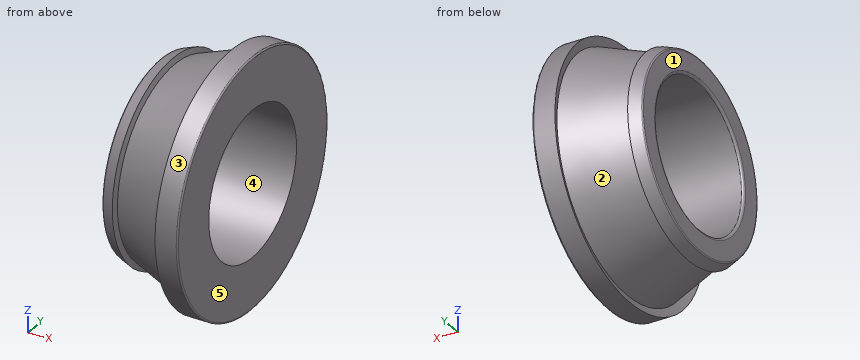
Solid Edge part; units mm, degrees
sketch "Sketch1" plane through (0, 0, 0) normal (0, 0, 1) x (1, 0, 0)
  arc A0 (0, 15.5) -> (0.5, 15) centre (0.5, 15.5) ccw
  line L0 (0.5, 15) -> (19, 15)
  line L1 (19, 15) -> (19, 25.318)
  arc A1 (19, 25.318) -> (18.711, 25.607) centre (18.711, 25.318) ccw
  line L2 (18.711, 25.607) -> (14.373, 25.607)
  line L3 (14.373, 25.607) -> (15.0184, 23.853)
  line L4 (15.0184, 23.853) -> (2.95, 19.4124)
  line L5 (2.95, 19.4124) -> (2.5514, 20.4958)
  line L6 (2.5514, 20.4958) -> (0.1964, 19.6293)
  arc A2 (0.1964, 19.6293) -> (0, 19.3477) centre (0.3, 19.3477) ccw
  line L7 (0, 19.3477) -> (0, 15.5)
revolve "RevolvedProtrusion1" add sketch "Sketch1" angle 360 about axis through (50, 0, 0) along (-1, 0, 0)
Geometry check sheet. Reference: the model listing, model coordinates, mm. Face numbers are marked on the shaded views. A direction names the side the tool comes from. Coordinates: 2 decimals unless noted, no trailing zeros. Order: outer loops, then holes, each group sorted by start corner. A loop starts at its lowest first (then second) coordinate and runs counter-clockwise, first axis right, second up. Notation, with made-up numbers: (62.5, 74.5) - (94.5, 74.5) arc R23 ccw to (94.5, 94.5) - close; hole circle Ø4 at (87, 25.25). An arc over 180 degrees is marked (long way). Answer as a JSON object with one key per item and string values. Group by question number.
Item 1: Sectioned sample at D-D, the plane x = 16.75. Record the cut outline in (y, z), and give its area (3 significant figures).
Item 2: Sectioned sample at C-C, the plane x = 1.5. Record the cut outline in (y, z), and give its area (3 significant figures).
Item 3: Draft check along Z on the marked faces 3, 4 and 5. Enter one of: +Z half, -Z half, draft (parallel to the pull), parting line (faces both ways), or undercut.
Item 4: Tool access check on the marked faces 1 and 2. Record the directions out of +Z, -Z, +X, -X, +Y, -Y that give a thin tool (end or side, any length) a straight path to the whole face; none if there is none.
Item 5: Scan lines: probe 1 along Y at (x, z) = (12.75, 0); probe 2 along Z at (x, y) = (9.5, -5.5); probe 3 along Y at (x, z) = (13.75, 0). Record each from-to range of solid material in increasing order.
Item 6: Depth check by flat-ended pin: pin 1 Ø8 at (x, y) = (17, 3) entering from +Z; pin 2 Ø1 at (y, z) = (7, -13) entering from -X; pin 3 Ø1 at (x, y) = (16.5, 20.5) entering from -Z. Enter the tip coordinate at first touch or a pass-through.
Item 7: Sectioned sample at A-A, the plane y = 0. Record the cut outline in (x, z), and give its area (3 significant figures).
Resolved:
{
 "1": {"outline": "circle Ø51.21 at (0, 0); hole circle Ø30 at (0, 0)", "area": "1,350 mm^2"},
 "2": {"outline": "circle Ø40.22 at (0, 0); hole circle Ø30 at (0, 0)", "area": "564 mm^2"},
 "3": {"face 3": "parting line", "face 4": "undercut", "face 5": "draft"},
 "4": {"face 1": "+Z, -Z, -X, +Y, -Y", "face 2": "none"},
 "5": {"probe 1": "-23.02 to -15, 15 to 23.02", "probe 2": "-21.12 to -13.96, 13.96 to 21.12", "probe 3": "-23.39 to -15, 15 to 23.39"},
 "6": {"pin 1": "z = 25.61", "pin 2": "x = 0.06", "pin 3": "z = -15.99"},
 "7": {"outline": "(0, -19.35) arc R0.3 ccw to (0.2, -19.63) - (2.55, -20.5) - (2.95, -19.41) - (15.02, -23.85) - (14.37, -25.61) - (18.71, -25.61) arc R0.29 ccw to (19, -25.32) - (19, -15) - (0.5, -15) arc R0.5 ccw to (0, -15.5) - close; (0, 15.5) arc R0.5 ccw to (0.5, 15) - (19, 15) - (19, 25.32) arc R0.29 ccw to (18.71, 25.61) - (14.37, 25.61) - (15.02, 23.85) - (2.95, 19.41) - (2.55, 20.5) - (0.2, 19.63) arc R0.3 ccw to (0, 19.35) - close", "area": "275 mm^2"}
}
